Design review of the part built by this model. Coordinates are the model's own, in mm. Face numbers are marked on the shaded views. A direction names the side the tool comes from. Coordinates: 2 decimals unless noted, no trailing zeros. Write each loop counter-clockwise with the first axis right and the second up, starting at its lowest first coordinate (ties: lowest second). Pieces come first, ordered by that corner, then holes. Notation, with made-up numbers: (62.25, 45.5) - (102.25, 45.5) arc R13 cw to (102.25, 52.5) - close; hole circle Ø2 at (49.25, 77). An arc over 180 degrees is marked (long way). One line per item, written item: value.
from build123d import *

# Parameters (mm, degrees)
SKETCH1_R           = 30
BOSS_EXTRUDE1_DEPTH = 250
BOSS_EXTRUDE2_DEPTH = 100


with BuildPart() as part:
    # Sketch1 → Boss-Extrude1 (new body)
    with BuildSketch(Plane(origin=(0, 0, 0), x_dir=(1, 0, 0), z_dir=(0, 1, 0))):
        Circle(SKETCH1_R)
    extrude(amount=BOSS_EXTRUDE1_DEPTH)

    # Sketch3 → Boss-Extrude2 (add)
    with BuildSketch(Plane(origin=(0, 250, 0), x_dir=(1, 0, 0), z_dir=(0, 1, 0))):
        Polygon((-15, 0.769018566), (-15, 15), (15, 15), (15, -15), (-15, -15), align=None)
    extrude(amount=BOSS_EXTRUDE2_DEPTH)

    # Sketch4 → Revolve1 (revolve)
    with BuildSketch(Plane(origin=(0, 350, 0), x_dir=(1, 0, 0), z_dir=(0, 1, 0))):
        with BuildLine():
            Line((0, 8.5), (0, -8.5))
            ThreePointArc((0, -8.5), (8.5, 0), (0, 8.5))
        make_face()
    revolve(axis=Axis((0, 350, -8.5), (0, 0, 1)))


solid = part.part
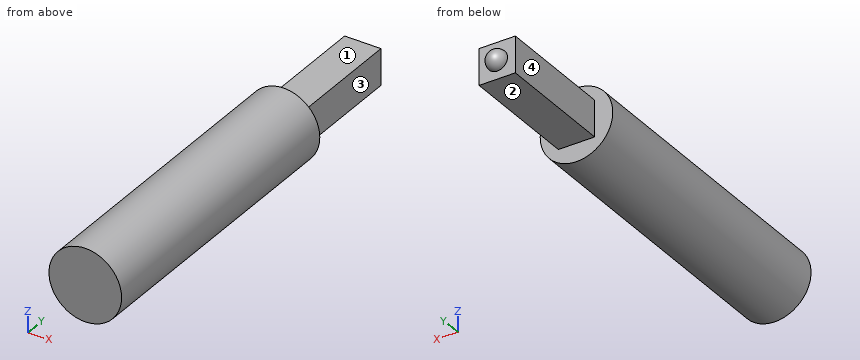
1. Consider section C-C, the plane y = 78. Write out the cut boundary in (x, z).
Answer block:
outline: circle Ø60 at (0, 0)
2. Consider section A-A, the plane x = 0. Write out the cut boundary in (y, z).
Answer block:
outline: (0, -30) - (250, -30) - (250, -15) - (350, -15) - (350, -8.5) arc R8.5 ccw to (350, 8.5) - (350, 15) - (250, 15) - (250, 30) - (0, 30) - close
3. Insertion check: pin 1 Ø4 at (x, y) = (8, 51.5) entering from +Z; pin 2 Ø3 at (y, z) = (235.5, -11) entering from +X; pin 3 Ø4 at (y, z) = (244, 1) entering from +X; pin 4 Ø24 at (y, z) = (279.5, -5.5) entering from +X. Each pin has a flat end and moves straight along its axis. Give the tip position at first contact, or say it passes through.
Answer block:
pin 1: stops at z = 29.39
pin 2: stops at x = 28.46
pin 3: stops at x = 30
pin 4: stops at x = 15
4. For the marked faces 1, 2, 3 and 4, list the 3-axis set-ups (+Z, -Z, +X, -X, +Y, -Y) from which the entire face can be reached by the end or side of a thin tool; tool diameter is ignored.
Answer block:
face 1: +Z, +X, -X, +Y
face 2: -Z, +X, -X, +Y
face 3: +Z, -Z, +X, +Y
face 4: +Z, -Z, -X, +Y
5. Consider section B-B, the plane z = 0. Write out the cut boundary in (x, y), then the cut area to 3 significant figures.
Answer block:
outline: (-30, 0) - (30, 0) - (30, 250) - (15, 250) - (15, 350) - (8.5, 350) arc R8.5 ccw to (-8.5, 350) - (-15, 350) - (-15, 250) - (-30, 250) - close
area: 18,100 mm^2
6. Consider section D-D, the plane z = -18. Write out the cut boundary in (x, y), then the cut area to 3 significant figures.
Answer block:
outline: (-24, 0) - (24, 0) - (24, 250) - (-24, 250) - close
area: 12,000 mm^2
7. Wall thickness on line 1 along Y through (x, z) = (10, -21.5); line 2 along X through (y, z) = (272, 0); line 3 along Y through (x, z) = (13.5, -7.5): over which ranges is each line inside the solid? List them lowest first.
Answer block:
line 1: y = 0 to 250
line 2: x = -15 to 15
line 3: y = 0 to 350
